```python
from build123d import *

# Parameters (mm, degrees)
SKETCH_1_R      = 2.1
EXTRUDE_1_DEPTH = 400


with BuildPart() as part:
    # 草图1 → 凸台-拉伸1 (new body)
    with BuildSketch(Plane.XY):
        Polygon((5.71, 20), (-5.71, 20), (-6.9, 18.81), (-6.9, 18.2), (-4.5, 18.2), (-4.5, 16.489949494), (-7.089949494, 13.9), (-12.910050506, 13.9), (-15.5, 16.489949494), (-15.5, 18.2), (-13.1, 18.2), (-13.1, 18.81), (-14.29, 20), (-20, 20), (-20, 14.29), (-18.81, 13.1), (-18.2, 13.1), (-18.2, 15.5), (-16.489949494, 15.5), (-13.9, 12.910050506), (-13.9, 7.089949494), (-16.489949494, 4.5), (-18.2, 4.5), (-18.2, 6.9), (-18.81, 6.9), (-20, 5.71), (-20, -5.71), (-18.81, -6.9), (-18.2, -6.9), (-18.2, -4.5), (-16.489949494, -4.5), (-13.9, -7.089949494), (-13.9, -12.910050506), (-16.489949494, -15.5), (-18.2, -15.5), (-18.2, -13.1), (-18.81, -13.1), (-20, -14.29), (-20, -20), (-14.29, -20), (-13.1, -18.81), (-13.1, -18.2), (-15.5, -18.2), (-15.5, -16.489949494), (-12.910050506, -13.9), (-7.089949494, -13.9), (-4.5, -16.489949494), (-4.5, -18.2), (-6.9, -18.2), (-6.9, -18.81), (-5.71, -20), (5.71, -20), (6.9, -18.81), (6.9, -18.2), (4.5, -18.2), (4.5, -16.489949494), (7.089949494, -13.9), (12.910050506, -13.9), (15.5, -16.489949494), (15.5, -18.2), (13.1, -18.2), (13.1, -18.81), (14.29, -20), (20, -20), (20, -14.29), (18.81, -13.1), (18.2, -13.1), (18.2, -15.5), (16.489949494, -15.5), (13.9, -12.910050506), (13.9, -7.089949494), (16.489949494, -4.5), (18.2, -4.5), (18.2, -6.9), (18.81, -6.9), (20, -5.71), (20, 5.71), (18.81, 6.9), (18.2, 6.9), (18.2, 4.5), (16.489949494, 4.5), (13.9, 7.089949494), (13.9, 12.910050506), (16.489949494, 15.5), (18.2, 15.5), (18.2, 13.1), (18.81, 13.1), (20, 14.29), (20, 20), (14.29, 20), (13.1, 18.81), (13.1, 18.2), (15.5, 18.2), (15.5, 16.489949494), (12.910050506, 13.9), (7.089949494, 13.9), (4.5, 16.489949494), (4.5, 18.2), (6.9, 18.2), (6.9, 18.81), align=None)
        with Locations((-10, 10)):
            Circle(SKETCH_1_R, mode=Mode.SUBTRACT)
        with Locations(Location((-10, -10, 0), (0, 0, 180))):
            Circle(SKETCH_1_R, mode=Mode.SUBTRACT)
        with Locations((10, -10)):
            Circle(SKETCH_1_R, mode=Mode.SUBTRACT)
        with Locations(Location((10, 10, 0), (0, 0, 180))):
            Circle(SKETCH_1_R, mode=Mode.SUBTRACT)
        Polygon((-6.1, 6.1), (-6.1, 12.910050506), (-3, 16.010050506), (-3, 18.2), (3, 18.2), (3, 16.010050506), (6.1, 12.910050506), (6.1, 6.1), (12.910050506, 6.1), (16.010050506, 3), (18.2, 3), (18.2, -3), (16.010050506, -3), (12.910050506, -6.1), (6.1, -6.1), (6.1, -12.910050506), (3, -16.010050506), (3, -18.2), (-3, -18.2), (-3, -16.010050506), (-6.1, -12.910050506), (-6.1, -6.1), (-12.910050506, -6.1), (-16.010050506, -3), (-18.2, -3), (-18.2, 3), (-16.010050506, 3), (-12.910050506, 6.1), align=None, mode=Mode.SUBTRACT)
    extrude(amount=EXTRUDE_1_DEPTH)


solid = part.part
```
Model file for the job. Use its own axes, mm. A direction names the side the tool comes from. Round coordinates to 2 decimals unless told otherwise and drop trailing zeros. Use CSV: the item, a comma, the result in double quotes. Start each with the question number.
Item 1: Band-saw the part on A-A (z = 205). State how many separate pieces and enclosed holes the cut face has, and give its area (3 significant figures).
Item 2: Tool access for faces 4 (the face through (-9, -6.1, 197)), 5 (the face through (-20, 0, 197)): list every direction of +Z, -Z, +X, -X, +Y, -Y with a clear straight run to the whole face (end or side of a thin tool).
Item 3: Pin check, flat tips, straight feed: P1, Ø10, axis at x = 2, y = 2.5, coming from the -Z side; P2, Ø1, axis at x = 11, z = 294.5, coming from the -Y side; P3, Ø4.5, axis at y = -10, z = 100, coming from the +X side; P4, Ø4.5, axis at y = 10.5, z = 190.5, coming from the -X side. Stop position of each tip, or through.
Item 4: Two-plate mould, pull along X, no slides. Class faces 1 (the face through (-6.1, 9, 197)), 2 (the face through (20, 0, 197)), 3 (the face through (-8, 8, 400)): released by +X, released by -X, zero draft, split by the parting line, or undercut.
Item 5: Drill centre lines: L1, parallel to X at y = 17.5, z = 297.5; L2, parallel to Y at x = -10, z = 213; L3, parallel to X at y = -2, z = 128. Where is each one in solid material? Low to high. Write a range as [from, to].
Checked values:
1,separate pieces,"1"
1,enclosed holes,"5"
1,area,"473 mm²"
2,face 4,"+Z, -Z"
2,face 5,"+Z, -Z, -X, +Y, -Y"
3,P1,"passes through"
3,P2,"stops at y = -13.9"
3,P3,"stops at x = 13.9"
3,P4,"stops at x = -13.9"
4,face 1,"undercut"
4,face 2,"released by +X"
4,face 3,"zero draft"
5,L1,"x = [-20, -15.5], [-4.5, -3], [3, 4.5], [15.5, 20]"
5,L2,"y = [-13.9, -12.1], [-7.9, -6.1], [6.1, 7.9], [12.1, 13.9]"
5,L3,"x = [-20, -18.2], [18.2, 20]"
